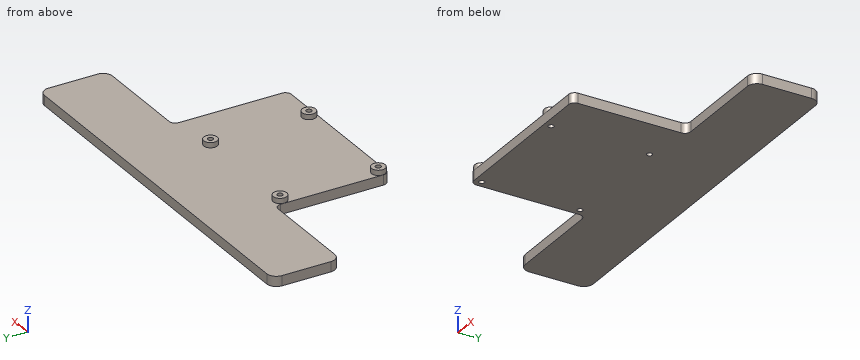
```python
from build123d import *

# Parameters (mm, degrees)
GRUNDFORM_R                     = 1.375
AUFSATZ_LINEAR_AUSTRAGEN1_DEPTH = 5
SKIZZE2_R                       = 3.375
SKIZZE2_R_2                     = 1.375
AUFSATZ_LINEAR_AUSTRAGEN2_DEPTH = 2.554396


with BuildPart() as part:
    # Grundform → Aufsatz-Linear austragen1 (new body)
    with BuildSketch(Plane.XY):
        with BuildLine():
            Line((-93.287044917, 40.781629135), (92.170661923, 40.781629135))
            ThreePointArc((92.170661923, 40.781629135), (95.523773437, 39.39272487), (96.912677703, 36.039613355))
            Line((96.912677703, 36.039613355), (96.912677703, 11.658797868))
            ThreePointArc((96.912677703, 11.658797868), (95.523773437, 8.305686353), (92.170661923, 6.916782087))
            Line((92.170661923, 6.916782087), (44.903892176, 6.916782087))
            ThreePointArc((44.903892176, 6.916782087), (42.782571833, 6.038102431), (41.903892176, 3.916782087))
            Line((41.903892176, 3.916782087), (41.903892176, -47.387842431))
            ThreePointArc((41.903892176, -47.387842431), (41.02521252, -49.509162775), (38.903892176, -50.387842431))
            Line((38.903892176, -50.387842431), (-40.02027517, -50.387842431))
            ThreePointArc((-40.02027517, -50.387842431), (-42.141595514, -49.509162775), (-43.02027517, -47.387842431))
            Line((-43.02027517, -47.387842431), (-43.02027517, 3.916782087))
            ThreePointArc((-43.02027517, 3.916782087), (-43.898954827, 6.038102431), (-46.02027517, 6.916782087))
            Line((-46.02027517, 6.916782087), (-93.287044917, 6.916782087))
            ThreePointArc((-93.287044917, 6.916782087), (-96.640156431, 8.305686353), (-98.029060697, 11.658797868))
            Line((-98.029060697, 11.658797868), (-98.029060697, 36.039613355))
            ThreePointArc((-98.029060697, 36.039613355), (-96.640156431, 39.39272487), (-93.287044917, 40.781629135))
        make_face()
        with Locations((-39.52027517, 2.112157569)):
            Circle(GRUNDFORM_R, mode=Mode.SUBTRACT)
        with Locations((18.47972483, 2.112157569)):
            Circle(GRUNDFORM_R, mode=Mode.SUBTRACT)
        with Locations((18.47972483, -46.887842431)):
            Circle(GRUNDFORM_R, mode=Mode.SUBTRACT)
        with Locations((-39.52027517, -46.887842431)):
            Circle(GRUNDFORM_R, mode=Mode.SUBTRACT)
    extrude(amount=AUFSATZ_LINEAR_AUSTRAGEN1_DEPTH)

    # Skizze2 → Aufsatz-Linear austragen2 (add)
    with BuildSketch(Plane.XY.offset(5)):
        with Locations((-39.52027517, 2.112157569)):
            Circle(SKIZZE2_R)
        with Locations((-39.52027517, 2.112157569)):
            Circle(SKIZZE2_R_2, mode=Mode.SUBTRACT)
        with Locations((18.47972483, 2.112157569)):
            Circle(SKIZZE2_R)
        with Locations((18.47972483, 2.112157569)):
            Circle(SKIZZE2_R_2, mode=Mode.SUBTRACT)
        with Locations((18.47972483, -46.887842431)):
            Circle(SKIZZE2_R)
        with Locations((18.47972483, -46.887842431)):
            Circle(SKIZZE2_R_2, mode=Mode.SUBTRACT)
        with Locations((-39.52027517, -46.887842431)):
            Circle(SKIZZE2_R)
        with Locations((-39.52027517, -46.887842431)):
            Circle(SKIZZE2_R_2, mode=Mode.SUBTRACT)
    extrude(amount=AUFSATZ_LINEAR_AUSTRAGEN2_DEPTH)


solid = part.part
```
For this review, take the finished solid that the model builds, in its own axes (mm). Give positions to 0.01 mm unless a question says otherwise; leave off trailing zeros. Order: outer loops, then holes, each group sorted by start corner. A loop starts at its lowest first (then second) coordinate and runs counter-clockwise, first axis right, second up.
1) Take a section at C-C (x = 25). Give the boundary of the cut face in (y, z).
2) Take a section at A-A (z = 2.25). Give the boundary of the cut face in (x, y) (3 decimals).
3) Take a section at B-B (y = 23.5). Give the boundary of the cut face in (x, z).
4) Wall thickness on line 1 (X direction, y = -29.5, z = 2.5); line 2 (Z direction, x = -34, y = 30); line 3 (X direction, y = 3, z = 2.5): over which ranges is each line inside the solid? List them lowest first.
5) Insertion check: pin 1 (1.5 mm diameter, centred on y = -21.5, z = 3, fed in from -X); pin 2 (12 mm diameter, centred on x = 65.5, y = 25.5, fed in from +Z); pin 3 (2 mm diameter, centred on y = -28.5, z = 2.5, fed in from +X). Each pin has a flat end and moves straight along its axis. Give the tip position at first contact, or say it passes through.
Derived:
1. outline: (-50.39, 0) - (40.78, 0) - (40.78, 5) - (-50.39, 5) - close
2. outline: (-98.029, 11.659) arc R4.742 ccw to (-93.287, 6.917) - (-46.02, 6.917) arc R3 cw to (-43.02, 3.917) - (-43.02, -47.388) arc R3 ccw to (-40.02, -50.388) - (38.904, -50.388) arc R3 ccw to (41.904, -47.388) - (41.904, 3.917) arc R3 cw to (44.904, 6.917) - (92.171, 6.917) arc R4.742 ccw to (96.913, 11.659) - (96.913, 36.04) arc R4.742 ccw to (92.171, 40.782) - (-93.287, 40.782) arc R4.742 ccw to (-98.029, 36.04) - close; hole circle Ø2.75 at (-39.52, -46.888); hole circle Ø2.75 at (-39.52, 2.112); hole circle Ø2.75 at (18.48, -46.888); hole circle Ø2.75 at (18.48, 2.112)
3. outline: (-98.03, 0) - (96.91, 0) - (96.91, 5) - (-98.03, 5) - close
4. line 1: x = -43.02 to 41.9
4. line 2: z = 0 to 5
4. line 3: x = -43.02 to -40.57, -38.47 to 17.43, 19.53 to 41.9
5. pin 1: stops at x = -43.02
5. pin 2: stops at z = 5
5. pin 3: stops at x = 41.9
